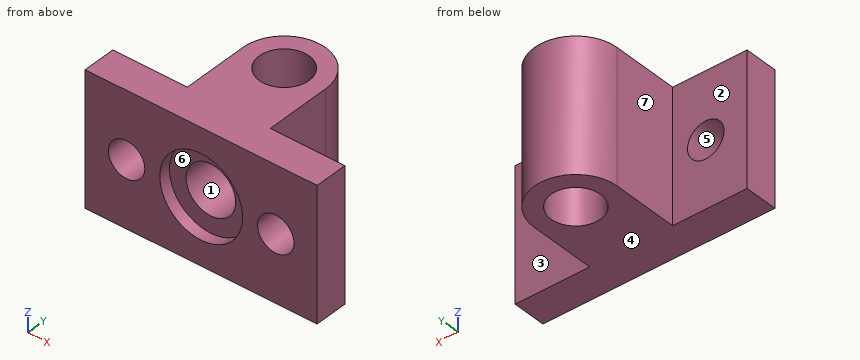
```python
from build123d import *

# Parameters (mm, degrees)
BASE_SKETCH_W                        = 14
BASE_SKETCH_H                        = 8
BASE_EXTRUDE_DEPTH                   = 2
PROTRUSION_EXTRUDE_REACH             = 6
PROTRUSION_SKETCH_W                  = 5
PROTRUSION_SKETCH_H                  = 4
PROTRUSION_EXTRUDE_DIRECTION_2_REACH = 6
F_3_0_3_DIAMETER_HOLE1_D             = 3
F_2_2_2_2_DIAMETER_HOLE1_D           = 2.2
F_3_0_3_DIAMETER_HOLE2_D             = 3
F_3_0_3_DIAMETER_HOLE2_DEPTH         = 6
F_3_0_3_DIAMETER_HOLE2_TIP           = 0.901290929
F_5MM_CUT_SKETCH_R                   = 2.5
F_5_MM_DIAMETER_CUT_DEPTH            = 0.7


with BuildPart() as part:
    # Base Sketch → Base Extrude (new body)
    with BuildSketch(Plane(origin=(0, 0, 0), x_dir=(1, 0, 0), z_dir=(0, 1, 0))):
        Rectangle(BASE_SKETCH_W, BASE_SKETCH_H)
    extrude(amount=BASE_EXTRUDE_DEPTH)

    # Protrusion Extrude: up to this face of the body (flat: up to its plane)
    protrusion_extrude_end = Plane(part.part.faces().sort_by_distance((0, 1, 4))[0])
    # Protrusion Sketch → Protrusion Extrude (add, up to the picked face)
    with BuildSketch(Plane.XY, mode=Mode.PRIVATE) as protrusion_extrude_sk1:
        with BuildLine():
            ThreePointArc((-2.5, 6), (0, 8.5), (2.5, 6))
            Line((2.5, 6), (-2.5, 6))
        make_face()
    protrusion_extrude_tool1 = split(extrude(protrusion_extrude_sk1.sketch, amount=PROTRUSION_EXTRUDE_REACH, mode=Mode.PRIVATE), bisect_by=protrusion_extrude_end, keep=Keep.BOTH, mode=Mode.PRIVATE)
    add(protrusion_extrude_tool1.solids().sort_by_distance((0, 7.061033, 0))[0])
    # Protrusion Sketch → Protrusion Extrude (add, up to the picked face)
    with BuildSketch(Plane.XY, mode=Mode.PRIVATE) as protrusion_extrude_sk2:
        with Locations((0, 4)):
            Rectangle(PROTRUSION_SKETCH_W, PROTRUSION_SKETCH_H)
    protrusion_extrude_tool2 = split(extrude(protrusion_extrude_sk2.sketch, amount=PROTRUSION_EXTRUDE_REACH, mode=Mode.PRIVATE), bisect_by=protrusion_extrude_end, keep=Keep.BOTH, mode=Mode.PRIVATE)
    add(protrusion_extrude_tool2.solids().sort_by_distance((0, 4, 0))[0])

    # Protrusion Extrude direction 2: up to this face of the body (flat: up to its plane)
    protrusion_extrude_direction_2_end = Plane(part.part.faces().sort_by_distance((0, 1, -4))[0])
    # Protrusion Sketch → Protrusion Extrude direction 2 (add, up to the picked face)
    with BuildSketch(Plane.XY, mode=Mode.PRIVATE) as protrusion_extrude_direction_2_sk1:
        with BuildLine():
            ThreePointArc((-2.5, 6), (0, 8.5), (2.5, 6))
            Line((2.5, 6), (-2.5, 6))
        make_face()
    protrusion_extrude_direction_2_tool1 = split(extrude(protrusion_extrude_direction_2_sk1.sketch, amount=-PROTRUSION_EXTRUDE_DIRECTION_2_REACH, mode=Mode.PRIVATE), bisect_by=protrusion_extrude_direction_2_end, keep=Keep.BOTH, mode=Mode.PRIVATE)
    add(protrusion_extrude_direction_2_tool1.solids().sort_by_distance((0, 7.061033, 0))[0])
    # Protrusion Sketch → Protrusion Extrude direction 2 (add, up to the picked face)
    with BuildSketch(Plane.XY, mode=Mode.PRIVATE) as protrusion_extrude_direction_2_sk2:
        with Locations((0, 4)):
            Rectangle(PROTRUSION_SKETCH_W, PROTRUSION_SKETCH_H)
    protrusion_extrude_direction_2_tool2 = split(extrude(protrusion_extrude_direction_2_sk2.sketch, amount=-PROTRUSION_EXTRUDE_DIRECTION_2_REACH, mode=Mode.PRIVATE), bisect_by=protrusion_extrude_direction_2_end, keep=Keep.BOTH, mode=Mode.PRIVATE)
    add(protrusion_extrude_direction_2_tool2.solids().sort_by_distance((0, 4, 0))[0])

    # Ø3.0 (3) Diameter Hole1 (through all)
    with Locations(Plane.XY.offset(4)):
        with Locations((0, 6)):
            Hole(F_3_0_3_DIAMETER_HOLE1_D / 2)

    # Ø2.2 (2.2) Diameter Hole1 (through all)
    with Locations(Plane(origin=(0, 0, 0), x_dir=(-1, 0, 0), z_dir=(0, -1, 0))):
        with Locations((4.5, 0), (-4.5, 0)):
            Hole(F_2_2_2_2_DIAMETER_HOLE1_D / 2)

    # Ø3.0 (3) Diameter Hole2
    with Locations(Plane(origin=(0, 0, 0), x_dir=(-1, 0, 0), z_dir=(0, -1, 0))):
        with Locations((0, 0)):
            Hole(F_3_0_3_DIAMETER_HOLE2_D / 2, depth=F_3_0_3_DIAMETER_HOLE2_DEPTH)
            with Locations((0, 0, -(F_3_0_3_DIAMETER_HOLE2_DEPTH + F_3_0_3_DIAMETER_HOLE2_TIP / 2))):  # 118° drill point
                Cone(0, F_3_0_3_DIAMETER_HOLE2_D / 2, F_3_0_3_DIAMETER_HOLE2_TIP, mode=Mode.SUBTRACT)

    # 5mm Cut Sketch → 5 mm diameter Cut (cut)
    with BuildSketch(Plane(origin=(0, 0, 0), x_dir=(1, 0, 0), z_dir=(0, 1, 0))):
        Circle(F_5MM_CUT_SKETCH_R)
    extrude(amount=F_5_MM_DIAMETER_CUT_DEPTH, mode=Mode.SUBTRACT)


solid = part.part
```
Check sheet for the modelled part. Datum: model origin and axes. Units: mm. Face numbers are marked on the shaded views. A direction names the side the tool comes from. Coordinates: 2 decimals unless noted, no trailing zeros. Loops run counter-clockwise (first coordinate to the right, second up) from the corner with the lowest first, then second, coordinate; pieces in that order, holes last.
1) Sectioned sample at D-D (y = 2.5). Record the boundary of the cut face in (x, z).
2) Sectioned sample at A-A (x = -4.5). Record the boundary of the cut face in (y, z).
3) Sectioned sample at B-B (x = 0). Record the boundary of the cut face in (y, z).
4) Gauge pin test, flat ends, axial feed: pin 1 (3.5 mm diameter, centred on x = 5, z = -2, fed in from +Y); pin 2 (2 mm diameter, centred on y = 3.5, z = 0, fed in from -X); pin 3 (3 mm diameter, centred on y = 7, z = -0.5, fed in from +X). Record the tip position at first contact, or that the pin passes through.
5) Release check for a two-part mould opening along X. For the marked faces 4, 5, 6 and 7 record: released by +X, released by -X, zero draft, split by the parting line, or undercut.
6) Access from +Z, -Z, +X, -X, +Y, -Y to the whole of each face (thin tool, end or side, straight path). Record for the marked faces 1, 2 and 3.
7) Sectioned sample at C-C (z = 2). Record the boundary of the cut face in (x, y).
8) Material ranges on probe 1 along X at (y, z) = (6, -1.5); probe 2 along Y at (x, z) = (0, -1.75); probe 3 along Z at (x, y) = (0, 2.3), recorded low to high.
Check sheet entries:
1. outline: (-2.5, -4) - (2.5, -4) - (2.5, 4) - (-2.5, 4) - close; hole circle Ø3 at (0, 0)
2. outline: (0, -4) - (2, -4) - (2, -1.1) - (0, -1.1) - close; (0, 1.1) - (2, 1.1) - (2, 4) - (0, 4) - close
3. outline: (0, -4) - (4.5, -4) - (4.5, -1.5) - (0.7, -1.5) - (0.7, -2.5) - (0, -2.5) - close; (0, 2.5) - (0.7, 2.5) - (0.7, 1.5) - (4.5, 1.5) - (4.5, 4) - (0, 4) - close; (7.5, -4) - (8.5, -4) - (8.5, 4) - (7.5, 4) - close
4. pin 1: stops at y = 2
4. pin 2: stops at x = -2.5
4. pin 3: stops at x = 2.5
5. face 4: zero draft
5. face 5: undercut
5. face 6: undercut
5. face 7: released by -X
6. face 1: -Y
6. face 2: +Z, -Z, -X, +Y
6. face 3: +Z, -Z, +X, +Y
7. outline: (-7, 0) - (-1.5, 0) - (-1.5, 0.7) - (1.5, 0.7) - (1.5, 0) - (7, 0) - (7, 2) - (2.5, 2) - (2.5, 6) arc R2.5 ccw to (-2.5, 6) - (-2.5, 2) - (-7, 2) - close; hole circle Ø3 at (0, 6)
8. probe 1: x = -2.5 to -1.5, 1.5 to 2.5
8. probe 2: y = 0.7 to 4.5, 7.5 to 8.5
8. probe 3: z = -4 to -1.5, 1.5 to 4
